The model under review builds one solid part; all positions refer to its coordinate system, in mm. Give positions to 0.01 mm unless a question says otherwise; leave off trailing zeros. Order: outer loops, then holes, each group sorted by start corner. A loop starts at its lowest first (then second) coordinate and runs counter-clockwise, first axis right, second up.
```python
from build123d import *

# Parameters (mm, degrees)
F0_W     = 48.6210244843
F0_H     = 48.6210244843
F0_R     = 2.15265
F1_DEPTH = 6.35
F6_W     = 2.794
F6_H     = 1.27
F8_R     = 0.2032


with BuildPart() as f1:
    # F0 (on Front) → F1 (new body)
    with BuildSketch(Plane.XZ):
        Rectangle(F0_W, F0_H)
        with Locations((-17.9605122421, -17.9605122421)):
            Circle(F0_R, mode=Mode.SUBTRACT)
        with Locations((17.9605122421, -17.9605122421)):
            Circle(F0_R, mode=Mode.SUBTRACT)
        with Locations((-17.9605122421, 17.9605122421)):
            Circle(F0_R, mode=Mode.SUBTRACT)
        with Locations((17.9605122421, 17.9605122421)):
            Circle(F0_R, mode=Mode.SUBTRACT)
    extrude(amount=F1_DEPTH)

    # F6 (on 3pt) → F7 (revolve, cut)
    with BuildSketch(Plane(origin=(0, 0, 0), x_dir=(1, 0, 0), z_dir=(0, 0, -1))):
        with Locations((-19.7993, 0.635)):
            Rectangle(F6_W, F6_H)
    revolve(axis=Axis((0, 0.4501026124, 0), (0, -1, 0)), mode=Mode.SUBTRACT)

    # F8
    f8_edges = [f1.edges().sort_by_distance(p)[0] for p in [
        (21.1963, -1.27, 0),
        (18.4023, 0, 0),
    ]]
    fillet(f8_edges, radius=F8_R)


solid = f1.part
```
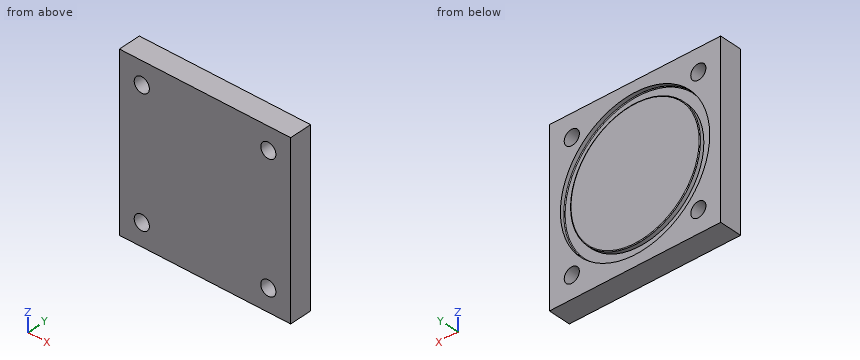
Item 1: For line 1 (Z direction, x = 0, y = -0.5); line 2 (Z direction, x = -18, y = -5); line 3 (X direction, y = -0.5, z = 2), list the stretches that pass through material, from the lowest coordinate up.
Values found:
line 1: z = -24.31 to -21.2, -18.4 to 18.4, 21.2 to 24.31
line 2: z = -24.31 to -20.11, -15.81 to 15.81, 20.11 to 24.31
line 3: x = -24.31 to -21.1, -18.29 to 18.29, 21.1 to 24.31
Item 2: Take a section at A-A (x = 0). Give the boundary of the cut face in (y, z).
Values found:
outline: (-6.35, -24.31) - (0, -24.31) - (0, -21.2) - (-1.07, -21.2) arc R0.2 cw to (-1.27, -20.99) - (-1.27, -18.4) - (-0.2, -18.4) arc R0.2 ccw to (0, -18.2) - (0, 18.2) arc R0.2 ccw to (-0.2, 18.4) - (-1.27, 18.4) - (-1.27, 20.99) arc R0.2 cw to (-1.07, 21.2) - (0, 21.2) - (0, 24.31) - (-6.35, 24.31) - close
Item 3: Take a section at C-C (z = 0). Give the boundary of the cut face in (x, y), and give its area (3 significant figures).
Values found:
outline: (-24.31, -6.35) - (24.31, -6.35) - (24.31, 0) - (21.2, 0) - (21.2, -1.07) arc R0.2 cw to (20.99, -1.27) - (18.4, -1.27) - (18.4, -0.2) arc R0.2 ccw to (18.2, 0) - (-18.2, 0) arc R0.2 ccw to (-18.4, -0.2) - (-18.4, -1.27) - (-20.99, -1.27) arc R0.2 cw to (-21.2, -1.07) - (-21.2, 0) - (-24.31, 0) - close
area: 302 mm2
Item 4: Take a section at B-B (y = -4.5). Give the boundary of the cut face in (x, z), and give its area (3 significant figures).
Values found:
outline: (-24.31, -24.31) - (24.31, -24.31) - (24.31, 24.31) - (-24.31, 24.31) - close; hole circle Ø4.31 at (-17.96, -17.96); hole circle Ø4.31 at (-17.96, 17.96); hole circle Ø4.31 at (17.96, -17.96); hole circle Ø4.31 at (17.96, 17.96)
area: 2,310 mm2
